```python
from build123d import *

# Parameters (mm, degrees)
MODEL_R                  = 1.8
RESSALTO_EXTRUS_O1_DEPTH = 6


with BuildPart() as part:
    # Model → Ressalto-extrusão1 (new body)
    with BuildSketch(Plane.XY):
        Polygon((64.544232036, 102.085333217), (58.944232036, 102.085333217), (58.944232036, 110.085333217), (53.944232036, 110.085333217), (35.344232036, 56.085333217), (35.344232036, 51.085333217), (29.744232036, 51.085333217), (29.485412991, 51.051259043), (29.244232036, 50.95135862), (29.037125255, 50.792439998), (28.878206632, 50.585333217), (28.77830621, 50.344152262), (28.744232036, 50.085333217), (28.744232036, 45.485333217), (28.77830621, 45.226514172), (28.878206632, 44.985333217), (29.037125255, 44.778226435), (29.244232036, 44.619307813), (29.485412991, 44.51940739), (29.744232036, 44.485333217), (35.344232036, 44.485333217), (35.344232036, 39.202796806), (44.344232036, 39.202796806), (44.344232036, 44.985333217), (50.944232036, 44.985333217), (50.944232036, 21.485333217), (44.344232036, 21.485333217), (44.344232036, 24.197608641), (29.744232036, 24.197608641), (29.485412991, 24.163534467), (29.244232036, 24.063634044), (29.037125255, 23.904715422), (28.878206632, 23.697608641), (28.77830621, 23.456427686), (28.744232036, 23.197608641), (28.744232036, 12.285333217), (28.77830621, 12.026514172), (28.878206632, 11.785333217), (29.037125255, 11.578226435), (29.244232036, 11.419307813), (29.485412991, 11.31940739), (29.744232036, 11.285333217), (35.344232036, 11.285333217), (35.344232036, 7.387063336), (44.340453402, 7.387063336), (44.344232036, 12.190525094), (50.944232036, 12.185333217), (50.940455526, 7.387063336), (58.944232036, 7.387063336), (58.944232036, 12.585333217), (64.544232036, 12.585333217), (64.803051081, 12.61940739), (65.044232036, 12.719307813), (65.251338817, 12.878226435), (65.41025744, 13.085333217), (65.510157862, 13.326514172), (65.544232036, 13.585333217), (65.544232036, 21.585333217), (65.510157862, 21.844152262), (65.41025744, 22.085333217), (65.251338817, 22.292439998), (65.044232036, 22.45135862), (64.803051081, 22.551259043), (64.544232036, 22.585333217), (58.944232036, 22.585333217), (58.944232036, 38.085333217), (64.544232036, 38.085333217), (64.803051081, 38.11940739), (65.044232036, 38.219307813), (65.251338817, 38.378226435), (65.41025744, 38.585333217), (65.510157862, 38.826514172), (65.544232036, 39.085333217), (65.544232036, 47.085333217), (65.510157862, 47.344152262), (65.41025744, 47.585333217), (65.251338817, 47.792439998), (65.044232036, 47.95135862), (64.803051081, 48.051259043), (64.544232036, 48.085333217), (58.944232036, 48.085333217), (58.944232036, 92.085333217), (64.544232036, 92.085333217), (64.803051081, 92.11940739), (65.044232036, 92.219307813), (65.251338817, 92.378226435), (65.41025744, 92.585333217), (65.510157862, 92.826514172), (65.544232036, 93.085333217), (65.544232036, 101.085333217), (65.510157862, 101.344152262), (65.41025744, 101.585333217), (65.251338817, 101.792439998), (65.044232036, 101.95135862), (64.803051081, 102.051259043), align=None)
        with Locations((39.844232036, 52.085333217)):
            Circle(MODEL_R, mode=Mode.SUBTRACT)
        Polygon((43.944232036, 19.069932909), (39.844232036, 21.437069013), (35.744232036, 19.069932909), (35.744232036, 14.335660702), (39.844232036, 11.968524598), (43.944232036, 14.335660702), align=None, mode=Mode.SUBTRACT)
    extrude(amount=RESSALTO_EXTRUS_O1_DEPTH)


solid = part.part
```
Part model, mm, in its own coordinate system. A direction names the side the tool comes from. Round coordinates to 2 decimals unless told otherwise and drop trailing zeros. Loops run counter-clockwise (first coordinate to the right, second up) from the corner with the lowest first, then second, coordinate; pieces in that order, holes last.
Item 1: Drop flat-ended pins along their axis: P1, Ø1.5, axis at y = 27, z = 3.5, coming from the -X side; P2, Ø1.2, axis at y = 9.5, z = 3, coming from the -X side; P3, Ø3, axis at y = 106, z = 3, coming from the +X side. Give the stop position or say it passes through.
Item 2: Cut at D-D, the plane x = 53. Give the cut face in (y, z).
Item 3: Cut at A-A, the plane y = 18. Give the cut face in (x, z).
Item 4: Drill centre lines: line 1 (Y direction, x = 59.5, z = 5.15); line 2 (X direction, y = 15, z = 4.35); line 3 (Y direction, x = 34, z = 2.8). Where is each one in solid material? Low to high.
Item 5: Mould opens along Y. For faces 1 (the face through (35.744, 17, 3)), 2 (the face through (40, 7.387, 3)), 3 (the face through (58.944, 106, 3)) say: +Y half, -Y half, draft (parallel to the pull), parting line (faces both ways), or undercut.
Item 6: 3-axis set-ups, long thin cutter, end or side, ignore diameter. For faces 4 (the face through (50.944, 33, 3)), 5 (the face through (40, 39.203, 3)), 6 (the face through (28.744, 18, 3)), 7 (the face through (62, 92.085, 3)): which of +Z, -Z, +X, -X, +Y, -Y reach the whole face in a straight line?
Item 7: Cut at C-C, the plane y = 36.5. Give the cut face in (x, z), then the cut area to 3 significant figures.
Item 8: Cut at B-B, the plane x = 45.5. Give the cut face in (y, z), then the cut area to 3 significant figures.
A:
1. P1: stops at x = 50.94
1. P2: stops at x = 35.34
1. P3: stops at x = 58.94
2. outline: (7.39, 0) - (107.34, 0) - (107.34, 6) - (7.39, 6) - close
3. outline: (28.74, 0) - (35.74, 0) - (35.74, 6) - (28.74, 6) - close; (43.94, 0) - (65.54, 0) - (65.54, 6) - (43.94, 6) - close
4. line 1: y = 12.59 to 22.59, 38.09 to 48.09, 92.09 to 102.09
4. line 2: x = 28.74 to 35.74, 43.94 to 65.54
4. line 3: y = 11.29 to 24.2, 44.49 to 51.09
5. face 1: undercut
5. face 2: -Y half
5. face 3: draft
6. face 4: +Z, -Z
6. face 5: +Z, -Z, -X
6. face 6: +Z, -Z, -X, +Y, -Y
6. face 7: +Z, -Z, +X
7. outline: (50.94, 0) - (58.94, 0) - (58.94, 6) - (50.94, 6) - close
7. area: 48.0 mm2
8. outline: (12.19, 0) - (21.49, 0) - (21.49, 6) - (12.19, 6) - close; (44.99, 0) - (85.57, 0) - (85.57, 6) - (44.99, 6) - close
8. area: 299 mm2
